Design review of the part shown in the three views and the two pictorial views. Dimensions are in mm from the part's minimum x, y and z. A direction names the side the tool comes from. Give positions to 0.01 mm unless a question says otherwise; leave off trailing zeros. Order: outer loops, then holes, each group sorted by start corner. A loop starts at its lowest first (then second) coordinate and runs counter-clockwise, first axis right, second up. Notation, with made-up numbers: (30, 19.25) -> (71, 19.25) arc R13 ccw to (71, 39.25) -> close; hole circle Ø11 at (-2.5, 80). An arc over 180 degrees is marked (long way). Answer in a Markdown table with one row per item. Add a question column.
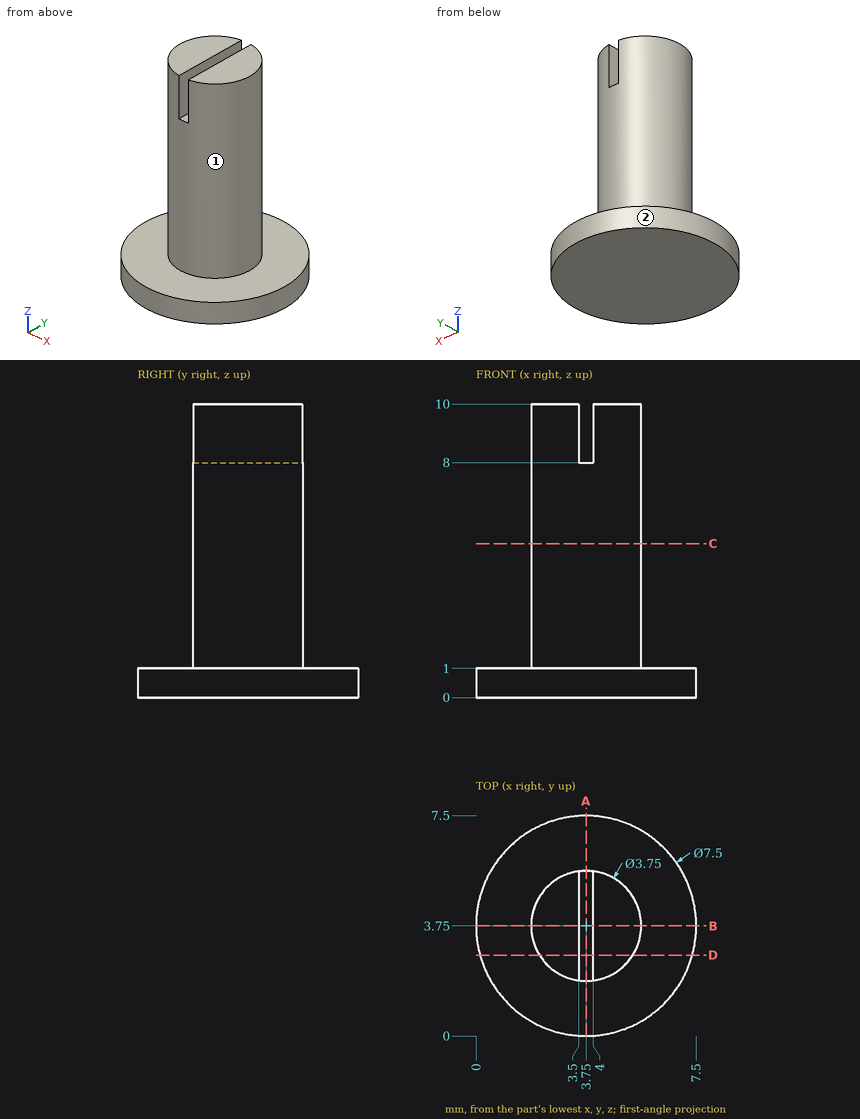
1) Add section D-D, the plane y = 2.75. Write out the cut boundary in (x, z).
2) Add section B-B, the plane y = 3.75. Write out the cut boundary in (x, z) (3 decimals), and give its area (4 significant figures).
3) Machinability: for the marked faces 1 and 2, which of the approach directions +Z, -Z, +X, -X, +Y, -Y give a long, thin tool a straight path to every point of the face, cutting with its end or side? Answer none if there is none.
4) Add section C-C, the plane z = 5.25. Write out the cut boundary in (x, y) (3 decimals).
5) Add section A-A, the plane x = 3.75. Write out the cut boundary in (y, z) (3 decimals), and give its area (4 significant figures).
6) For L1, parallel to Z at x = 5.25, y = 7; L2, parallel to Y at x = 3, z = 7; L3, parallel to X at y = 4.25, z = 4.25, list the stretches that pass through material, from the lowest coordinate up.
7) Clearance check with flat-ended pins moving along their axes: P1, Ø4, axis at x = 6, z = 2.5, coming from the -Y side; P2, Ø4, axis at x = 4.5, z = 4, coming from the -Y side (3 decimals); P3, Ø0.6, axis at y = 4.5, z = 9, coming from the +X side. State where each tip first meets the part, or that it passes through.
Verdict:
| question | item | result |
|---|---|---|
| 1 | outline | (0.14, 0) -> (7.36, 0) -> (7.36, 1) -> (5.34, 1) -> (5.34, 10) -> (4, 10) -> (4, 8) -> (3.5, 8) -> (3.5, 10) -> (2.16, 10) -> (2.16, 1) -> (0.14, 1) -> close |
| 2 | outline | (0, 0) -> (7.5, 0) -> (7.5, 1) -> (5.625, 1) -> (5.625, 10) -> (4, 10) -> (4, 8) -> (3.5, 8) -> (3.5, 10) -> (1.875, 10) -> (1.875, 1) -> (0, 1) -> close |
| 2 | area | 40.25 mm2 |
| 3 | face 1 | +Z |
| 3 | face 2 | +Z, -Z |
| 4 | outline | circle Ø3.75 at (3.75, 3.75) |
| 5 | outline | (0, 0) -> (7.5, 0) -> (7.5, 1) -> (5.625, 1) -> (5.625, 8) -> (1.875, 8) -> (1.875, 1) -> (0, 1) -> close |
| 5 | area | 33.75 mm2 |
| 6 | L1 | z = 0 to 1 |
| 6 | L2 | y = 2.03 to 5.47 |
| 6 | L3 | x = 1.94 to 5.56 |
| 7 | P1 | stops at y = 0.12 |
| 7 | P2 | stops at y = 1.875 |
| 7 | P3 | stops at x = 5.57 |
